Geometry: see drawing. Coordinates: mm, zero at the bounding-box minimum. A direction names the side the tool comes from. Coordinates: 2 decimals unless noted, no trailing zeros. Order: outer loops, then holes, each group sorted by start corner. A loop starts at its lowest first (then second) coordinate and runs counter-clockwise, first axis right, second up. Notation, with made-up numbers: (-27, 37.5) -> (-22, 37.5) arc R17 ccw to (-22, 62.5) -> close; hole circle Ø9 at (-29, 82). An arc over 180 degrees is marked (long way). Use one line per item in the form item = value.
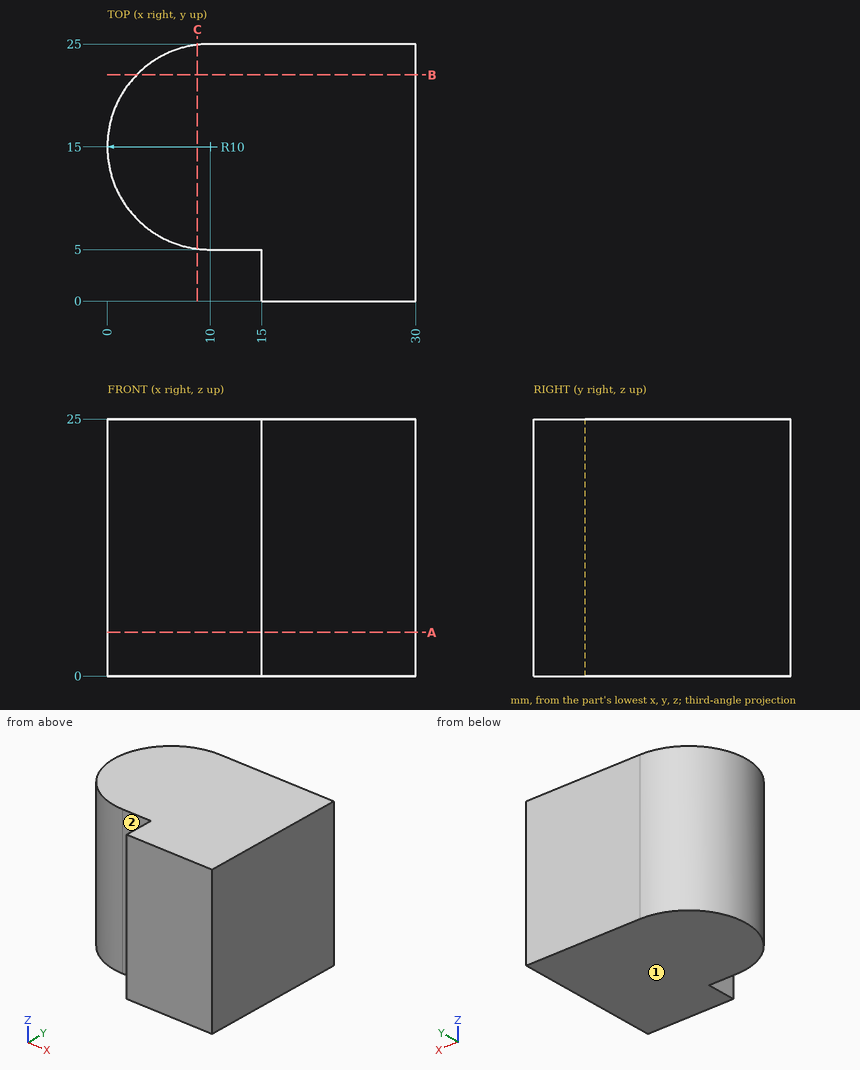
1) Contact query for flat-ended pins moving along their axis: P1, Ø4, axis at y = 20.5, z = 22.5, coming from the -X side; P2, Ø5.5, axis at x = 12, z = 10.5, coming from the -Y side. Output: stop coordinate, or through.
Results found:
P1 = 0.63
P2 = 5
2) Section C-C, the plane x = 8.75. Output: boundary loops of the cut face in (y, z), and give its area (3 significant figures).
Results found:
outline = (5.08, 0) -> (24.92, 0) -> (24.92, 25) -> (5.08, 25) -> close
area = 496 mm2
3) Section A-A, the plane z = 4.25. Output: boundary loops of the cut face in (x, y).
Results found:
outline = (10, 5) -> (15, 5) -> (15, 0) -> (30, 0) -> (30, 25) -> (10, 25) arc R10 ccw to start
4) Section B-B, the plane y = 22. Output: boundary loops of the cut face in (x, z).
Results found:
outline = (2.86, 0) -> (30, 0) -> (30, 25) -> (2.86, 25) -> close
5) Material intervals for probe 1 along X at (y, z) = (14.75, 7.25); probe 2 along X at (y, z) = (3.75, 12.75); probe 3 along Y at (x, z) = (4, 16.5), sorted ascending. Write a range as from..to.
Results found:
probe_1 = 0..30
probe_2 = 15..30
probe_3 = 7..23
6) Access query for the marked faces 1 and 2. Directions: +Z, -Z, +X, -X, +Y, -Y. A direction counts if a zero-diameter tool reaches every point of the face in a straight line with its end or side. Return the directions, or none.
Results found:
face_1 = -Z, +X, -X, +Y, -Y
face_2 = +Z, -Z, -X, -Y
